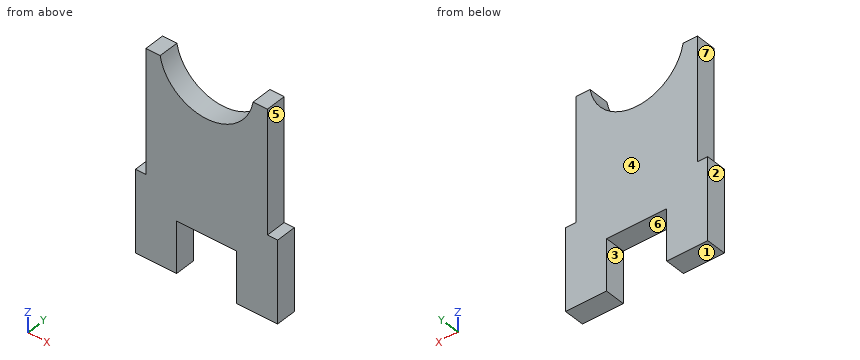
from build123d import *

# Parameters (mm, degrees)
F1_DEPTH = 12.7


with BuildPart() as f1:
    # F0 (on Front) → F1 (new body)
    with BuildSketch(Plane.XZ):
        with BuildLine():
            Line((-44.45, 76.2), (-44.45, 25.4))
            Line((-44.45, 25.4), (-19.05, 25.4))
            Line((-19.05, 25.4), (-19.05, 57.15))
            Line((-19.05, 57.15), (18.207463, 57.15))
            Line((18.207463, 57.15), (18.207463, 25.4))
            Line((18.207463, 25.4), (43.607463, 25.4))
            Line((43.607463, 25.4), (43.607463, 76.2))
            Line((43.607463, 76.2), (37.257463, 76.2))
            Line((37.257463, 76.2), (37.257463, 152.4))
            Line((37.257463, 152.4), (28.367463, 152.4))
            ThreePointArc((28.367463, 152.4), (-0.421268, 128.132977), (-29.21, 152.4))
            Line((-29.21, 152.4), (-38.1, 152.4))
            Line((-38.1, 152.4), (-38.1, 76.2))
            Line((-38.1, 76.2), (-44.45, 76.2))
        make_face()
    extrude(amount=F1_DEPTH)


solid = f1.part
Could you check a few things on this model? Use its own coordinates, in mm. Face numbers are marked on the shaded views. A direction names the side the tool comes from. Round coordinates to 2 decimals unless told otherwise and drop trailing zeros. Order: outer loops, then holes, each group sorted by start corner. A loop starts at its lowest first (then second) coordinate and runs counter-clockwise, first axis right, second up. Notation, with made-up numbers: M -14.5,-19 L 26.5,-19 A15 ccw 26.5,0 Z; hole C 57.25,-6 d7. An arc over 180 degrees is marked long. One line per item, written item: value.
(1) Imagine slicing it at B-B (y = -8). Write out the boundary of the cut face in (x, z).
Ans:
outline: M -44.45,25.4 L -19.05,25.4 L -19.05,57.15 L 18.21,57.15 L 18.21,25.4 L 43.61,25.4 L 43.61,76.2 L 37.26,76.2 L 37.26,152.4 L 28.37,152.4 A29.21 cw -29.21,152.4 L -38.1,152.4 L -38.1,76.2 L -44.45,76.2 Z
(2) Imagine slicing it at C-C (z = 99). Write out the boundary of the cut face in (x, y), and give its area (3 significant figures).
Ans:
outline: M -38.1,-12.7 L 37.26,-12.7 L 37.26,0 L -38.1,0 Z
area: 957 mm^2
(3) If we mould it in two halves opening along X, with no side actions, what happens to the marked faces 1, 2 and 3? For each: released by +X, released by -X, zero draft, split by the parting line, or undercut.
Ans:
face 1: zero draft
face 2: released by -X
face 3: undercut
(4) I need wall thicknesses on line 1 along X through (y, z) = (-11.75, 39); line 2 along X through (y, z) = (-1, 116); line 3 along X through (y, z) = (-3, 130.5). Which ranges of each line are inside material? Lowest first, please. Write a range as from..to.
Ans:
line 1: x = -44.45..-19.05, 18.21..43.61
line 2: x = -38.1..37.26
line 3: x = -38.1..-11.94, 11.1..37.26
(5) Which directions (+Z, -Z, +X, -X, +Y, -Y) give clear straight access to the entire face, cutting with the end or side of a thin tool? Please do the marked faces 4, 5, 6 and 7.
Ans:
face 4: +Z, -Z, +X, -X, +Y
face 5: +Z, +X, +Y, -Y
face 6: -Z, +Y, -Y
face 7: +Z, -X, +Y, -Y
(6) Imagine slicing it at D-D (x = 23.5). Write out the boundary of the cut face in (y, z).
Ans:
outline: M -12.7,25.4 L 0,25.4 L 0,140.58 L -12.7,140.58 Z
(7) I'm going to push flat-ended pins straight in: P1, Ø2, axis at x = -11, y = -9, coming from the +Z side; P2, Ø6.5, axis at y = -6.5, z = 105.5, coming from the -X side; P3, Ø4, axis at y = -5, z = 95.5, coming from the +X side. Where does each tip first touch, or does it pass through?
Ans:
P1: stops at z = 130.53
P2: stops at x = -38.1
P3: stops at x = 37.26
(8) Imagine slicing it at A-A (z = 43.5). Write out the boundary of the cut face in (x, y).
Ans:
outline: M -44.45,-12.7 L -19.05,-12.7 L -19.05,0 L -44.45,0 Z; M 18.21,-12.7 L 43.61,-12.7 L 43.61,0 L 18.21,0 Z
